```python
from build123d import *

# Parameters (mm, degrees)
SKETCH1_R               = 34
BOSS_EXTRUDE1_DEPTH     = 10
SKETCH2_R               = 19.7871926
SKETCH2_R_2             = 2
CUT_EXTRUDE1_DEPTH      = 10
SKETCH3_R               = 4.837531333
SKETCH4_W               = 4.837531333
SKETCH4_H               = 4.837531333
CUT_EXTRUDE3_DEPTH      = 38
CUT_EXTRUDE3_DEPTH_BACK = 38
SKETCH5_W               = 72.361656805
SKETCH5_H               = 8.896778435
BOSS_EXTRUDE2_START     = 35
SKETCH6_R               = 22.2871926
SKETCH6_R_2             = 19.7871926
BOSS_EXTRUDE2_DEPTH     = 35
SKETCH7_R               = 21.0371926
SKETCH7_R_2             = 19.7871926
CUT_EXTRUDE4_DEPTH      = 25
CUT_EXTRUDE5_DEPTH      = 59
CUT_EXTRUDE5_DEPTH_BACK = 45
SKETCH9_R               = 2


with BuildPart() as part:
    # Sketch1 → Boss-Extrude1 (new body)
    with BuildSketch(Plane(origin=(0, 0, 0), x_dir=(1, 0, 0), z_dir=(0, 1, 0))):
        with Locations(Location((0, 0, 0), (0, 0, 270))):
            Circle(SKETCH1_R)
    extrude(amount=BOSS_EXTRUDE1_DEPTH)

    # Sketch2 → Cut-Extrude1 (cut)
    with BuildSketch(Plane.XZ):
        with Locations(Location((0, 0, 0), (0, 0, 270))):
            Circle(SKETCH2_R)
        with Locations(Location((-22.1, 12.5, 0), (0, 0, 270))):
            Circle(SKETCH2_R_2)
        with Locations(Location((22.1, 12.5, 0), (0, 0, 90))):
            Circle(SKETCH2_R_2)
        with Locations(Location((22.1, -12.5, 0), (0, 0, 270))):
            Circle(SKETCH2_R_2)
        with Locations(Location((-22.1, -12.5, 0), (0, 0, 90))):
            Circle(SKETCH2_R_2)
    extrude(amount=-CUT_EXTRUDE1_DEPTH, mode=Mode.SUBTRACT)

    # Sketch3 → Cut-Revolve1 (revolve, cut)
    with BuildSketch(Plane(origin=(0, 0, 0), x_dir=(0, 0, -1), z_dir=(1, 0, 0)), mode=Mode.PRIVATE) as cut_revolve1_sk:
        with Locations((-34, 5)):
            Circle(SKETCH3_R)
    revolve(cut_revolve1_sk.sketch.rotate(Axis((0, 0, 0), (0, 1, 0)), 180), axis=Axis((0, 0, 0), (0, 1, 0)), mode=Mode.SUBTRACT)

    # Sketch4 → Cut-Revolve2 (revolve, cut)
    with BuildSketch(Plane(origin=(0, 0, 0), x_dir=(0, 0, -1), z_dir=(1, 0, 0)), mode=Mode.PRIVATE) as cut_revolve2_sk:
        with Locations((-31.581234333, 2.581234333)):
            Rectangle(SKETCH4_W, SKETCH4_H)
    revolve(cut_revolve2_sk.sketch.rotate(Axis((0, 0, 0), (0, 1, 0)), 180), axis=Axis((0, 0, 0), (0, 1, 0)), mode=Mode.SUBTRACT)

    # Sketch5 → Cut-Extrude3 (cut, two sides: drawn at the far end of the back side and taken through both)
    with BuildSketch(Plane(origin=(0, 0, 0), x_dir=(0, 0, -1), z_dir=(1, 0, 0)).offset(-CUT_EXTRUDE3_DEPTH_BACK)):
        with Locations((-0.901301775, 0.551610782)):
            Rectangle(SKETCH5_W, SKETCH5_H)
    extrude(amount=CUT_EXTRUDE3_DEPTH + CUT_EXTRUDE3_DEPTH_BACK, mode=Mode.SUBTRACT)

    # Sketch6 → Boss-Extrude2 (add)
    with BuildSketch(Plane.XZ.offset(-5).offset(BOSS_EXTRUDE2_START)):
        with Locations(Location((0, 0, 0), (0, 0, 270))):
            Circle(SKETCH6_R)
        with Locations(Location((0, 0, 0), (0, 0, 270))):
            Circle(SKETCH6_R_2, mode=Mode.SUBTRACT)
    extrude(amount=-BOSS_EXTRUDE2_DEPTH)

    # Sketch7 → Cut-Extrude4 (cut)
    with BuildSketch(Plane.XZ.offset(30)):
        with Locations(Location((0, 0, 0), (0, 0, 270))):
            Circle(SKETCH7_R)
        with Locations(Location((0, 0, 0), (0, 0, 270))):
            Circle(SKETCH7_R_2, mode=Mode.SUBTRACT)
    extrude(amount=-CUT_EXTRUDE4_DEPTH, mode=Mode.SUBTRACT)

    # Sketch9 → Cut-Extrude5 (cut, two sides: drawn at the far end of the back side and taken through both)
    with BuildSketch(Plane(origin=(0, 0, 0), x_dir=(0, 0, -1), z_dir=(1, 0, 0)).offset(-CUT_EXTRUDE5_DEPTH_BACK)):
        with Locations(Location((0, -17.5, 0), (0, 0, 180))):
            Circle(SKETCH9_R)
    extrude(amount=CUT_EXTRUDE5_DEPTH + CUT_EXTRUDE5_DEPTH_BACK, mode=Mode.SUBTRACT)


solid = part.part
```
Here's how the part is built. I have some questions about the finished solid (model axes, mm). A direction names the side the tool comes from. Give positions to 0.01 mm unless a question says otherwise; leave off trailing zeros. Loops run counter-clockwise (first coordinate to the right, second up) from the corner with the lowest first, then second, coordinate; pieces in that order, holes last. Notation, with made-up numbers: M 45.25,-5 L 90.25,-5 A29 cw 90.25,20 Z; hole C 53,53 d11. An arc over 180 degrees is marked long. Use one line per item in the form item = value. Start each with the question number.
Q1. If we section it at B-B (x = 0): Write out the boundary of the cut face in (y, z).
Q2. I need wall thicknesses on line 1 along Y through (x, z) = (22, 0); line 2 along Y through (x, z) = (10.5, -20); line 3 along X through (y, z) = (-18, -5). Which ranges of each line are inside material? Lowest first, please.
Q3. Which directions (+Z, -Z, +X, -X, +Y, -Y) give clear straight access to the entire face, cutting with the end or side of a thin tool? Please do faces 4 (the cylindrical face through (-20.537, -17.675, 4.56)), 5 (the cylindrical face through (-21.624, -17.588, -1.998)).
Q4. Will these pins go through, and if not, where does the flat tip stop? pin 1 Ø3.5 at (x, z) = (22.1, 12.5) entering from -Y; pin 2 Ø3 at (y, z) = (-5.5, 0.5) entering from +X; pin 3 Ø5 at (y, z) = (-17.5, 0) entering from -X; pin 4 Ø10 at (y, z) = (4, 3) entering from +X.
Q5. If we section it at D-D (y = -26.5): Write out the boundary of the cut face in (x, z).
Q6. Thinking about a two-plate mould opening in Z: for faces 1 (the cylindrical face through (21.605, -18.101, 1.908)), 2 (the flat face through (-8, -30, -20)), 3 (the cylindrical face through (22.098, -12.745, 2.901)), which applies, +Z half, -Z half, draft (parallel to the pull), parting line (faces both ways), or undercut?
Q7. If we section it at A-A (z = 0): Write out the boundary of the cut face in (x, y).
Taken from the geometry:
q1.outline = M -30,-22.29 L 5,-22.29 L 5,-29.16 A4.84 cw 9.84,-34 L 10,-34 L 10,-19.79 L -5,-19.79 L -5,-21.04 L -30,-21.04 Z; M -30,21.04 L -5,21.04 L -5,19.79 L 10,19.79 L 10,34 L 9.84,34 A4.84 cw 5,29.16 L 5,22.29 L -30,22.29 Z
q2.line_1 = -30 to -19.5, -15.5 to 10
q2.line_2 = 5 to 10
q2.line_3 = -21.72 to -20.43, 20.43 to 21.72
q3.face_4 = -Y
q3.face_5 = +X, -X
q4.pin_1 = through
q4.pin_2 = 22.29
q4.pin_3 = -22.29
q4.pin_4 = 31.15
q5.outline = C 0,0 d44.57; hole C 0,0 d42.07
q6.face_1 = undercut
q6.face_2 = draft
q6.face_3 = parting line
q7.outline = M -34,9.84 A4.84 cw -29.16,5 L -22.29,5 L -22.29,-15.5 L -21.04,-15.5 L -21.04,-5 L -19.79,-5 L -19.79,10 L -34,10 Z; M -22.29,-30 L -21.04,-30 L -21.04,-19.5 L -22.29,-19.5 Z; M 19.79,-5 L 21.04,-5 L 21.04,-15.5 L 22.29,-15.5 L 22.29,5 L 29.16,5 A4.84 cw 34,9.84 L 34,10 L 19.79,10 Z; M 21.04,-30 L 22.29,-30 L 22.29,-19.5 L 21.04,-19.5 Z
